from build123d import *

# Parameters (mm, degrees)
SKETCH_1_W             = 240
SKETCH_1_H             = 100
EXTRUDE_1_DEPTH        = 6
SKETCH_2_R             = 1.55
CUT_EXTRUDE_1_DEPTH    = 261.069221555
SKETCH_3_W             = 60
SKETCH_3_H             = 15
CUT_EXTRUDE_2_DEPTH    = 261.069221555
SKETCH_4_W             = 30
SKETCH_4_H             = 80
CUT_EXTRUDE_3_DEPTH    = 261.069221555
SKETCH_5_R             = 3
CUT_EXTRUDE_4_DEPTH    = 3
EXTRUDE_3_DEPTH        = 240
CUT_EXTRUDE_5_DEPTH    = 10
CUT_EXTRUDE_6_DEPTH    = 10
PATTERN_LINEAR_1_COUNT = 23
PATTERN_LINEAR_1_PITCH = 10
CUT_EXTRUDE_7_DEPTH    = 10
CUT_EXTRUDE_8_DEPTH    = 261.376650259


with BuildPart() as part:
    # 草图1 → 凸台-拉伸1 (new body)
    with BuildSketch(Plane(origin=(0, 0, 0), x_dir=(0, 0, -1), z_dir=(1, 0, 0))):
        with Locations((120, -50)):
            Rectangle(SKETCH_1_W, SKETCH_1_H)
    extrude(amount=EXTRUDE_1_DEPTH)

    # 草图2 → 切除-拉伸1 (cut, through all)
    with BuildSketch(Plane(origin=(6, 0, 0), x_dir=(0, 0, -1), z_dir=(1, 0, 0))):
        with Locations((8, -54)):
            Circle(SKETCH_2_R)
        with Locations((45, -80)):
            Circle(SKETCH_2_R)
        with Locations((45, -54)):
            Circle(SKETCH_2_R)
        with Locations((8, -80)):
            Circle(SKETCH_2_R)
        with Locations(Location((232, -80, 0), (0, 0, 180))):
            Circle(SKETCH_2_R)
        with Locations(Location((195, -54, 0), (0, 0, 180))):
            Circle(SKETCH_2_R)
        with Locations(Location((195, -80, 0), (0, 0, 180))):
            Circle(SKETCH_2_R)
        with Locations(Location((232, -54, 0), (0, 0, 180))):
            Circle(SKETCH_2_R)
    extrude(amount=-CUT_EXTRUDE_1_DEPTH, mode=Mode.SUBTRACT)

    # 草图3 → 切除-拉伸2 (cut, through all)
    with BuildSketch(Plane(origin=(6, 0, 0), x_dir=(0, 0, -1), z_dir=(1, 0, 0))):
        with Locations((40, -27.5)):
            Rectangle(SKETCH_3_W, SKETCH_3_H)
        with Locations((200, -27.5)):
            Rectangle(SKETCH_3_W, SKETCH_3_H)
    extrude(amount=-CUT_EXTRUDE_2_DEPTH, mode=Mode.SUBTRACT)

    # 草图4 → 切除-拉伸3 (cut, through all)
    with BuildSketch(Plane(origin=(6, 0, 0), x_dir=(0, 0, -1), z_dir=(1, 0, 0))):
        with Locations((100, -50)):
            Rectangle(SKETCH_4_W, SKETCH_4_H)
        with Locations((140, -50)):
            Rectangle(SKETCH_4_W, SKETCH_4_H)
    extrude(amount=-CUT_EXTRUDE_3_DEPTH, mode=Mode.SUBTRACT)

    # 草图5 → 切除-拉伸4 (cut)
    with BuildSketch(Plane.ZY):
        with Locations((-195, -80)):
            Circle(SKETCH_5_R)
        with Locations((-232, -80)):
            Circle(SKETCH_5_R)
        with Locations((-195, -54)):
            Circle(SKETCH_5_R)
        with Locations((-232, -54)):
            Circle(SKETCH_5_R)
        with Locations((-45, -80)):
            Circle(SKETCH_5_R)
        with Locations((-8, -80)):
            Circle(SKETCH_5_R)
        with Locations((-8, -54)):
            Circle(SKETCH_5_R)
        with Locations((-45, -54)):
            Circle(SKETCH_5_R)
    extrude(amount=-CUT_EXTRUDE_4_DEPTH, mode=Mode.SUBTRACT)

    # 草图8 → 凸台-拉伸3 (add)
    with BuildSketch(Plane(origin=(0, 0, -240), x_dir=(-1, 0, 0), z_dir=(0, 0, -1))):
        Polygon((-6, 0), (-14, 4.618802154), (-14, 16.618802154), (-8, 16.618802154), (-8, 4.618802154), (0, 0), align=None)
    extrude(amount=-EXTRUDE_3_DEPTH)

    # 草图9 → 切除-拉伸5 (cut)
    with BuildSketch(Plane(origin=(14, 0, 0), x_dir=(0, 0, -1), z_dir=(1, 0, 0))):
        Polygon((0, 16.618802154), (0, 10.618802154), (5, 16.618802154), align=None)
    extrude(amount=-CUT_EXTRUDE_5_DEPTH, mode=Mode.SUBTRACT)

    # 草图10 → 切除-拉伸6 (cut)
    with BuildSketch(Plane(origin=(14, 0, 0), x_dir=(0, 0, -1), z_dir=(1, 0, 0))):
        Polygon((5, 16.618802154), (10, 10.618802154), (15, 16.618802154), align=None)
    cut_extrude_6 = extrude(amount=-CUT_EXTRUDE_6_DEPTH, mode=Mode.SUBTRACT)

    # 阵列(线性)1: 切除-拉伸6 ×23
    with Locations(*[(0, 0, -i * PATTERN_LINEAR_1_PITCH) for i in range(1, PATTERN_LINEAR_1_COUNT)]):
        add(cut_extrude_6, mode=Mode.SUBTRACT)

    # 草图11 → 切除-拉伸7 (cut)
    with BuildSketch(Plane(origin=(14, 0, 0), x_dir=(0, 0, -1), z_dir=(1, 0, 0))):
        Polygon((235, 16.618802154), (240, 10.618802154), (240, 16.618802154), align=None)
    extrude(amount=-CUT_EXTRUDE_7_DEPTH, mode=Mode.SUBTRACT)

    # 草图12 → 切除-拉伸8 (cut, through all)
    with BuildSketch(Plane(origin=(0, 0, -240), x_dir=(-1, 0, 0), z_dir=(0, 0, -1))):
        Polygon((-14, 7.618802154), (-12.5, 16.618802154), (-14, 16.618802154), align=None)
        Polygon((-9.5, 16.618802154), (-8, 7.618802154), (-8, 16.618802154), align=None)
    extrude(amount=-CUT_EXTRUDE_8_DEPTH, mode=Mode.SUBTRACT)


solid = part.part
Work out the finished part from the listing and answer in its coordinate system (mm). A direction names the side the tool comes from. Round coordinates to 2 decimals unless told otherwise and drop trailing zeros. Order: outer loops, then holes, each group sorted by start corner. A loop starts at its lowest first (then second) coordinate and runs counter-clockwise, first axis right, second up. Notation, with made-up numbers: M 9.25,20 L 17.25,20 A26 cw 17.25,40 Z; hole C -36.5,-12.75 d2. An arc over 180 degrees is marked long. One line per item, written item: value.
Q1. Flat-ended cylindrical pins translate along their axes: pin 1 (1.9 mm diameter, centred on y = -80, z = -8, fed in from +X); pin 2 (7 mm diameter, centred on y = -80, z = -8, fed in from +X); pin 3 (2 mm diameter, centred on x = 10, z = -58.5, fed in from -Y); pin 4 (1.5 mm diameter, centred on x = 3, z = -182, fed in from +Y). Find the tip coordinate at first contact, or state that the pin passes through.
Derived:
pin 1: through
pin 2: x = 6
pin 3: y = 1.73
pin 4: y = 2.17
Q2. Find section B-B on y = -7. Write down the section's boundary in (x, z).
Derived:
outline: M 0,-240 L 6,-240 L 6,0 L 0,0 Z
Q3. For faces 1 (the face through (4.056, 2.342, -121.68)), 2 (the face through (11.035, 13.577, -232.465)), 3 (the face through (3, -20, -200)), 4 (the face through (6, -49, -118)), 5 (the face through (4, -44, 0)), determine the directions among +Z, -Z, +X, -X, +Y, -Y from which every point of the face is accessible in a straight line to the end or side of a thin tool.
Derived:
face 1: +Z, -Z, -X, +Y
face 2: +X, -X, +Y
face 3: +X, -X
face 4: +Z, -Z, +X, -Y
face 5: +Z, +X, -X, +Y, -Y
Q4. Find section A-A on y = -39. Write down the section's boundary in (x, z).
Derived:
outline: M 0,-240 L 6,-240 L 6,-155 L 0,-155 Z; M 0,-125 L 6,-125 L 6,-115 L 0,-115 Z; M 0,-85 L 6,-85 L 6,0 L 0,0 Z
Q5. Determine the mould class of faces 6 (the face through (1.48, -82.93, -8.65)), 7 (the face through (4, -44, -240)), 8 (the face through (11.035, 13.661, -167.465)) for opening direction Y: released by +Y, released by -Y, zero draft, split by the parting line, or undercut.
Derived:
face 6: undercut
face 7: zero draft
face 8: released by +Y
Q6. Straight lines are drawn through the part: line 1 (Z direction, x = 3, y = -16); line 2 (Y direction, x = 5, z = -232); line 3 (Y direction, x = 4.6, z = -232). For each, find the intervals that lie inside material, in ascending order.
Derived:
line 1: -240 to -155, -125 to -115, -85 to 0
line 2: -100 to -81.55, -78.45 to -55.55, -52.45 to 2.89
line 3: -100 to -81.55, -78.45 to -55.55, -52.45 to 2.66
